Check sheet for the modelled part. Datum: model origin and axes. Units: mm. Face numbers are marked on the shaded views. A direction names the side the tool comes from. Round coordinates to 2 decimals unless told otherwise and drop trailing zeros. Write each loop counter-clockwise with the first axis right and the second up, starting at its lowest first coordinate (ties: lowest second). Pieces come first, ordered by that corner, then holes. Notation, with made-up numbers: (49, 87.5) -> (74, 87.5) arc R19 cw to (74, 123.5) -> close; hole circle Ø8 at (73, 83.5). An arc over 180 degrees is marked (long way). Put each result on its own line as item: value. Start each with the question number.
from build123d import *

# Parameters (mm, degrees)
SKETCH1_W           = 37.3
SKETCH1_H           = 19.3
SKETCH1_R           = 2
BOSS_EXTRUDE1_DEPTH = 1.25
BOSS_EXTRUDE2_DEPTH = 1.25
BOSS_EXTRUDE3_START = -18.05
BOSS_EXTRUDE3_DEPTH = 1.25
SKETCH3_R           = 12.5
BOSS_EXTRUDE4_DEPTH = 16.8


with BuildPart() as part:
    # Sketch1 → Boss-Extrude1 (new body)
    with BuildSketch(Plane(origin=(0, 0, 0), x_dir=(1, 0, 0), z_dir=(0, 1, 0))):
        Rectangle(SKETCH1_W, SKETCH1_H)
        with Locations(Location((-14.5, 0, 0), (0, 0, 270))):
            Circle(SKETCH1_R, mode=Mode.SUBTRACT)
        with Locations(Location((14.5, 0, 0), (0, 0, 90))):
            Circle(SKETCH1_R, mode=Mode.SUBTRACT)
    extrude(amount=BOSS_EXTRUDE1_DEPTH)

    # Sketch2 → Boss-Extrude2 (add)
    with BuildSketch(Plane.XY.offset(9.65)):
        with BuildLine():
            Line((-14.15, 0), (14.15, 0))
            Line((14.15, 0), (2.704926778, -23.860753361))
            ThreePointArc((2.704926778, -23.860753361), (0, -25.563305432), (-2.704926778, -23.860753361))
            Line((-2.704926778, -23.860753361), (-14.15, 0))
        make_face()
    extrude(amount=-BOSS_EXTRUDE2_DEPTH)

    # Sketch2<2> → Boss-Extrude3 (add)
    with BuildSketch(Plane.XY.offset(9.65).offset(BOSS_EXTRUDE3_START)):
        with BuildLine():
            Line((-14.15, 0), (14.15, 0))
            Line((14.15, 0), (2.704926778, -23.860753361))
            ThreePointArc((2.704926778, -23.860753361), (0, -25.563305432), (-2.704926778, -23.860753361))
            Line((-2.704926778, -23.860753361), (-14.15, 0))
        make_face()
    extrude(amount=-BOSS_EXTRUDE3_DEPTH)

    # Sketch3 → Boss-Extrude4 (add)
    with BuildSketch(Plane(origin=(0, 0, 8.4), x_dir=(-1, 0, 0), z_dir=(0, 0, -1))):
        with Locations(Location((0, -22.563305432, 0), (0, 0, 129.511758747))):
            Circle(SKETCH3_R)
    extrude(amount=BOSS_EXTRUDE4_DEPTH)


solid = part.part
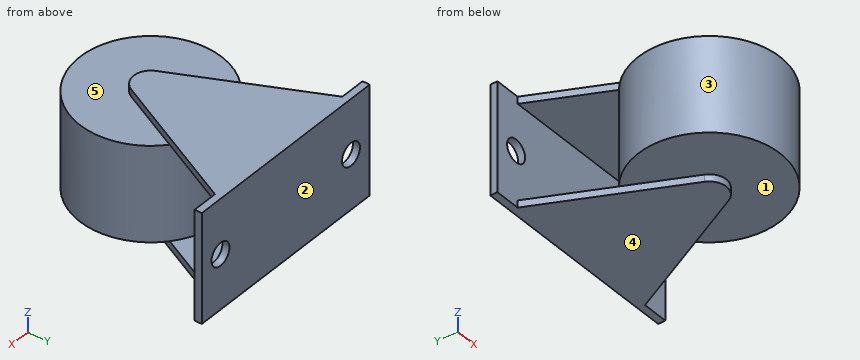
1. Material ranges on L1, parallel to X at y = 0.6, z = 0; L2, parallel to Z at x = -6.5, y = -4; L3, parallel to Z at x = 14.5, y = 1, recorded low to high. Write a range as [from, to].
2. Section check C-C, the plane x = -13.5. Enter the section's corners in (y, z), then the cut area to 3 significant figures.
3. Gauge pin test, flat ends, axial feed: P1, Ø10, axis at y = -31, z = 5, coming from the +X side; P2, Ø6, axis at y = -25.5, z = 2.5, coming from the -X side; P3, Ø2, axis at y = -31, z = 7.5, coming from the -X side. Record the tip position at first contact, or that the pin passes through.
4. Access from +Z, -Z, +X, -X, +Y, -Y to the whole of each face (thin tool, end or side, straight path). Record for the marked faces 4 and 5.
5. Section check B-B, the plane x = 0. Enter the section's corners in (y, z).
6. Section check A-A, the plane y = -1.5. Enter the section's corners in (x, z), then the cut area to 3 significant figures.
7. Section check D-D, the plane z = 0. Enter the section's corners in (x, y), then the cut area to 4 significant figures.
8. Draft check along Y on the marked faces 1, 2 and 3. Enter one of: released by +Y, released by -Y, zero draft, split by the parting line, or undercut.
Reply:
1. L1: x = [-18.65, -16.5], [-12.5, 12.5], [16.5, 18.65]
1. L2: z = [-9.65, -8.4], [8.4, 9.65]
1. L3: z = [-9.65, -2], [2, 9.65]
2. outline: (-1.36, -9.65) -> (1.25, -9.65) -> (1.25, -1.73) -> (0, -1.73) -> (0, -8.4) -> (-1.36, -8.4) -> close; (-1.36, 8.4) -> (0, 8.4) -> (0, 1.73) -> (1.25, 1.73) -> (1.25, 9.65) -> (-1.36, 9.65) -> close
2. area: 23.2 mm2
3. P1: stops at x = 12.02
3. P2: stops at x = -12.5
3. P3: stops at x = -10.05
4. face 4: -Z, +X, -X, +Y, -Y
4. face 5: +Z, -Y
5. outline: (-35.06, -8.4) -> (-25.56, -8.4) -> (-25.56, -9.65) -> (1.25, -9.65) -> (1.25, 9.65) -> (-25.56, 9.65) -> (-25.56, 8.4) -> (-35.06, 8.4) -> close; hole (-10.06, -8.4) -> (0, -8.4) -> (0, 8.4) -> (-10.06, 8.4) -> close
6. outline: (-13.43, -9.65) -> (13.43, -9.65) -> (13.43, -8.4) -> (-13.43, -8.4) -> close; (-13.43, 8.4) -> (13.43, 8.4) -> (13.43, 9.65) -> (-13.43, 9.65) -> close
6. area: 67.2 mm2
7. outline: (-18.65, 0) -> (-16.5, 0) -> (-16.5, 1.25) -> (-18.65, 1.25) -> close; circle Ø25 at (0, -22.56); (-12.5, 0) -> (12.5, 0) -> (12.5, 1.25) -> (-12.5, 1.25) -> close; (16.5, 0) -> (18.65, 0) -> (18.65, 1.25) -> (16.5, 1.25) -> close
7. area: 527.5 mm2
8. face 1: zero draft
8. face 2: released by +Y
8. face 3: undercut
